For this review, take the finished solid that the model builds, in its own axes (mm). A direction names the side the tool comes from. Coordinates: 2 decimals unless noted, no trailing zeros. Loops run counter-clockwise (first coordinate to the right, second up) from the corner with the lowest first, then second, coordinate; pieces in that order, holes last.
1. Take a section at A-A, the plane x = 0. State the section outline as (y, z) points, then the cut area to 3 significant figures.
2. Take a section at D-D, the plane y = 22.5. State the section outline as (x, z) points, then the cut area to 3 significant figures.
3. To check wall thickness, follow probe 1 along Y at (x, z) = (0, 3.35); probe 2 along Y at (x, z) = (-2.5, 1.8); probe 3 along Z at (x, y) = (14.5, 19.5). State the ranges of each line that lie inside material, in increasing order.
4. Machinability: for faces 4 (the face through (-13.887, -10.648, 3.493)), 5 (the face through (-8, 12, 4)), which of the approach directions +Z, -Z, +X, -X, +Y, -Y give a long, thin tool a straight path to every point of the face, cutting with its end or side? Answer none if there is none.
5. Mouldability with a two-part tool opening along Y and no side actions: class faces 1 (the face through (-20.3, -15.6, 0.5)), 2 (the face through (-6, -19, 1)), 3 (the face through (12.932, -5.362, 3.493)) as pulls with the +Y half, pulls with the -Y half, needs draft (parallel to the pull), parting line crosses it, or undercut.
6. Clearance check with flat-ended pins moving along their axes: P1, Ø22.5, axis at x = 0, y = 0, coming from the -Z side; P2, Ø1.5, axis at y = 0.5, z = 3, coming from the -X side; P3, Ø8, axis at x = 20, y = -8.5, coming from the +Z side; P4, Ø1.5, axis at x = -13.5, z = 0.5, coming from the -Y side. State where each tip first meets the part, or that it passes through.
7. Take a section at C-C, the plane x = -21.5. State the section outline as (y, z) points.
```python
from build123d import *

# Parameters (mm, degrees)
SKETCH_1_R      = 25.6
SKETCH_1_R_2    = 14
EXTRUDE_1_DEPTH = 1
SKETCH_2_R      = 17.5
SKETCH_2_R_2    = 14
EXTRUDE_2_DEPTH = 3
FILLET_2_R      = 2
FILLET_3_R      = 3


with BuildPart() as part:
    # 草图1 → 凸台-拉伸1 (new body)
    with BuildSketch(Plane.XY):
        Circle(SKETCH_1_R)
        Circle(SKETCH_1_R_2, mode=Mode.SUBTRACT)
    extrude(amount=EXTRUDE_1_DEPTH)

    # 草图2 → 凸台-拉伸2 (add)
    with BuildSketch(Plane.XY.offset(1)):
        Circle(SKETCH_2_R)
        Circle(SKETCH_2_R_2, mode=Mode.SUBTRACT)
    extrude(amount=EXTRUDE_2_DEPTH)

    # 圆角2
    fillet_2_edges = [part.edges().sort_by_distance(p)[0] for p in [
        (-17.5, 0, 1),
    ]]
    fillet(fillet_2_edges, radius=FILLET_2_R)

    # 圆角3
    fillet_3_edges = [part.edges().sort_by_distance(p)[0] for p in [
        (-14, 0, 0),
    ]]
    fillet(fillet_3_edges, radius=FILLET_3_R)


solid = part.part
```
Results list:
1. outline: (-25.6, 0) - (-17, 0) arc R3 ccw to (-14, 3) - (-14, 4) - (-17.5, 4) - (-17.5, 3) arc R2 cw to (-19.5, 1) - (-25.6, 1) - close; (14, 3) arc R3 ccw to (17, 0) - (25.6, 0) - (25.6, 1) - (19.5, 1) arc R2 cw to (17.5, 3) - (17.5, 4) - (14, 4) - close
1. area: 42.1 mm2
2. outline: (-12.21, 0) - (12.21, 0) - (12.21, 1) - (-12.21, 1) - close
2. area: 24.4 mm2
3. probe 1: y = -17.5 to -14, 14 to 17.5
3. probe 2: y = -17.72 to -14.03, 14.03 to 17.72
3. probe 3: z = 0 to 1
4. face 4: +Z
4. face 5: +Z, +X, -X, +Y, -Y
5. face 1: parting line crosses it
5. face 2: needs draft
5. face 3: undercut
6. P1: passes through
6. P2: stops at x = -17.64
6. P3: stops at z = 2.07
6. P4: stops at y = -22.2
7. outline: (-13.9, 0) - (13.9, 0) - (13.9, 1) - (-13.9, 1) - close
